Geometry: final body of the model. Coordinates: model frame, mm. Face numbers are marked on the shaded views. A direction names the side the tool comes from. Coordinates: 2 decimals unless noted, no trailing zeros. Loops run counter-clockwise (first coordinate to the right, second up) from the corner with the lowest first, then second, coordinate; pieces in that order, holes last. Notation, with made-up numbers: (52, -22.5) - (89, -22.5) arc R20 cw to (89, -16.5) - close; hole circle Ø10 at (-0.5, 28.25). An arc over 180 degrees is marked (long way). Answer in a Markdown table with one row per item.
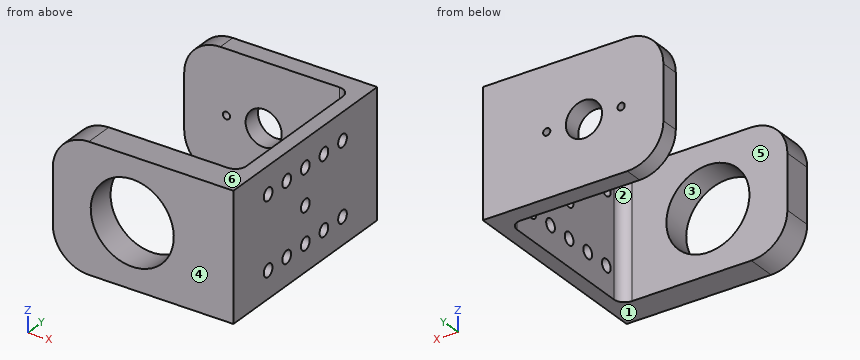
from build123d import *

# Parameters (mm, degrees)
SKETCH1_W           = 50
SKETCH1_H           = 35
SKETCH1_R           = 11.5
BOSS_EXTRUDE1_DEPTH = 8
SKETCH2_W           = 4
SKETCH2_H           = 35
BOSS_EXTRUDE2_DEPTH = 45
SKETCH3_W           = 50
SKETCH3_H           = 35
SKETCH3_R           = 5
SKETCH3_R_2         = 1
BOSS_EXTRUDE3_DEPTH = 5
FILLET1_R           = 10
FILLET2_R           = 3
SKETCH4_R           = 1.75
CUT_EXTRUDE1_DEPTH  = 79.550938887


with BuildPart() as part:
    # Sketch1 → Boss-Extrude1 (new body)
    with BuildSketch(Plane(origin=(0, 0, 0), x_dir=(1, 0, 0), z_dir=(0, 1, 0))):
        with Locations((3, 0)):
            Rectangle(SKETCH1_W, SKETCH1_H)
        with Locations(Location((0, 0, 0), (0, 0, 270))):
            Circle(SKETCH1_R, mode=Mode.SUBTRACT)
    extrude(amount=BOSS_EXTRUDE1_DEPTH)

    # Sketch2 → Boss-Extrude2 (add)
    with BuildSketch(Plane(origin=(0, 8, 0), x_dir=(1, 0, 0), z_dir=(0, 1, 0))):
        with Locations((26, 0)):
            Rectangle(SKETCH2_W, SKETCH2_H)
    extrude(amount=BOSS_EXTRUDE2_DEPTH)

    # Sketch3 → Boss-Extrude3 (add)
    with BuildSketch(Plane(origin=(0, 53, 0), x_dir=(1, 0, 0), z_dir=(0, 1, 0))):
        with Locations((3, 0)):
            Rectangle(SKETCH3_W, SKETCH3_H)
        with Locations(Location((0, 0, 0), (0, 0, 270))):
            Circle(SKETCH3_R, mode=Mode.SUBTRACT)
        with Locations(Location((10.3, 0, 0), (0, 0, 270))):
            Circle(SKETCH3_R_2, mode=Mode.SUBTRACT)
        with Locations(Location((-10.3, 0, 0), (0, 0, 270))):
            Circle(SKETCH3_R_2, mode=Mode.SUBTRACT)
    extrude(amount=BOSS_EXTRUDE3_DEPTH)

    # Fillet1
    fillet1_edges = [part.edges().sort_by_distance(p)[0] for p in [
        (-22, 55.5, -17.5),
        (-22, 55.5, 17.5),
        (-22, 4, 17.5),
        (-22, 4, -17.5),
    ]]
    fillet(fillet1_edges, radius=FILLET1_R)

    # Fillet2
    fillet2_edges = [part.edges().sort_by_distance(p)[0] for p in [
        (24, 8, 0),
        (24, 53, 0),
    ]]
    fillet(fillet2_edges, radius=FILLET2_R)

    # Sketch4 → Cut-Extrude1 (cut, through all)
    with BuildSketch(Plane(origin=(28, 0, 0), x_dir=(0, 0, -1), z_dir=(1, 0, 0))):
        with Locations((-10, 36.5)):
            Circle(SKETCH4_R)
        with Locations((10, 21.5)):
            Circle(SKETCH4_R)
        with Locations((0, 29)):
            Circle(SKETCH4_R)
        with Locations((-10, 44)):
            Circle(SKETCH4_R)
        with Locations((-10, 14)):
            Circle(SKETCH4_R)
        with Locations((10, 14)):
            Circle(SKETCH4_R)
        with Locations((-10, 29)):
            Circle(SKETCH4_R)
        with Locations((10, 29)):
            Circle(SKETCH4_R)
        with Locations((-10, 21.5)):
            Circle(SKETCH4_R)
        with Locations((10, 36.5)):
            Circle(SKETCH4_R)
        with Locations((10, 44)):
            Circle(SKETCH4_R)
    extrude(amount=-CUT_EXTRUDE1_DEPTH, mode=Mode.SUBTRACT)


solid = part.part
(1) Ray query, probe 1 along Y at (x, z) = (27, -10); probe 2 along Y at (x, z) = (-16, -10); probe 3 along Y at (x, z) = (-1, -6). Return the intervals inside material, ascending.
Verdict:
| item | result |
|---|---|
| probe 1 | y = 0 to 12.25, 15.75 to 19.75, 23.25 to 27.25, 30.75 to 34.75, 38.25 to 42.25, 45.75 to 58 |
| probe 2 | y = 0 to 8, 53 to 58 |
| probe 3 | y = 53 to 58 |
(2) Cut plane B-B on x = 0. Output: boundary loops of the cut face in (y, z), then the cut area to 3 significant figures.
Verdict:
| item | result |
|---|---|
| outline | (0, -17.5) - (8, -17.5) - (8, -11.5) - (0, -11.5) - close; (0, 11.5) - (8, 11.5) - (8, 17.5) - (0, 17.5) - close; (53, -17.5) - (58, -17.5) - (58, -5) - (53, -5) - close; (53, 5) - (58, 5) - (58, 17.5) - (53, 17.5) - close |
| area | 221 mm² |
(3) Cut plane A-A on y = 54. Output: boundary loops of the cut face in (x, z), then the cut area to 3 significant figures.
Verdict:
| item | result |
|---|---|
| outline | (-22, -7.5) arc R10 ccw to (-12, -17.5) - (28, -17.5) - (28, 17.5) - (-12, 17.5) arc R10 ccw to (-22, 7.5) - close; hole circle Ø2 at (-10.3, 0); hole circle Ø10 at (0, 0); hole circle Ø2 at (10.3, 0) |
| area | 1,620 mm² |
(4) Pull-direction query (Y, two-part tool) for the marked faces 4, 5 and 6; classes: pulls with the +Y half, pulls with the -Y half, needs draft (parallel to the pull), parting line crosses it, or undercut.
Verdict:
| item | result |
|---|---|
| face 4 | pulls with the -Y half |
| face 5 | undercut |
| face 6 | needs draft |
(5) Cut plane C-C on z = 0. State how many separate pieces and enclosed holes the cut face has, then the cut area to 3 significant figures.
Verdict:
| item | result |
|---|---|
| separate pieces | 6 |
| enclosed holes | 0 |
| area | 566 mm² |
(6) Access query for the marked faces 1, 2 and 3. Directions: +Z, -Z, +X, -X, +Y, -Y. A direction counts if a zero-diameter tool reaches every point of the face in a straight line with its end or side. Return the directions, or none.
Verdict:
| item | result |
|---|---|
| face 1 | -Z, +X, -X, +Y, -Y |
| face 2 | +Z, -Z, -X |
| face 3 | -Y |
(7) First-contact query: pin 1 Ø2 at (y, z) = (21.5, 10) entering from +X; pin 2 Ø4.5 at (y, z) = (44, 10) entering from -X; pin 3 Ø4.5 at (y, z) = (36.5, 10) entering from +X; pin 4 Ø11.5 at (x, z) = (0, 0) entering from -Y. Flat tips, straight axial feed; report the tip coordinate or a pass-through.
Verdict:
| item | result |
|---|---|
| pin 1 | passes through |
| pin 2 | stops at x = 24 |
| pin 3 | stops at x = 28 |
| pin 4 | stops at y = 53 |
(8) Cut plane D-D on y = 21.5. Output: boundary loops of the cut face in (x, z).
Verdict:
| item | result |
|---|---|
| outline | (24, -17.5) - (28, -17.5) - (28, -11.75) - (24, -11.75) - close; (24, -8.25) - (28, -8.25) - (28, 8.25) - (24, 8.25) - close; (24, 11.75) - (28, 11.75) - (28, 17.5) - (24, 17.5) - close |
